from build123d import *

# Parameters (mm, degrees)
F0_R     = 1.5
F1_DEPTH = 13
F0_W     = 7.7
F0_H     = 40
F2_DEPTH = 15
F3_R     = 1.5
F4_DEPTH = 15.001
F5_DEPTH = 5
F6_SIZE  = 1.5


with BuildPart() as f1:
    # F0 (on Right) → F1 (new body)
    with BuildSketch(Plane.YZ):
        Polygon((0, 50), (0, 0), (15, 0), (15, 10), (7.3, 10), (7.3, 50), align=None)
        with Locations((7.5, 5)):
            Circle(F0_R, mode=Mode.SUBTRACT)
    extrude(amount=F1_DEPTH)

    # F0 (on Right) → F2 (join)
    with BuildSketch(Plane.YZ):
        Polygon((0, 50), (0, 0), (15, 0), (15, 10), (7.3, 10), (7.3, 50), align=None)
        with Locations((7.5, 5)):
            Circle(F0_R, mode=Mode.SUBTRACT)
        with Locations((11.15, 30)):
            Rectangle(F0_W, F0_H)
        with Locations((7.5, 5)):
            Circle(F0_R)
    extrude(amount=-F2_DEPTH)

    # F3 (on face) → F4 (cut, through all)
    with BuildSketch(Plane.XZ):
        with Locations((-10, 45)):
            Circle(F3_R)
        with Locations((-10, 5)):
            Circle(F3_R)
    extrude(amount=-F4_DEPTH, mode=Mode.SUBTRACT)

    # F3 (on face) → F5 (cut, symmetric)
    with BuildSketch(Plane.XZ):
        Polygon((-10.010564, 2.401945), (-7.7553, 3.691824), (-7.744737, 6.289879), (-9.989436, 7.598055), (-12.2447, 6.308176), (-12.255263, 3.710121), align=None)
        with Locations((-10, 5)):
            Circle(F3_R, mode=Mode.SUBTRACT)
        Polygon((-7.758047, 46.312877), (-10.016008, 47.598027), (-12.257961, 46.28515), (-12.241953, 43.687123), (-9.983992, 42.401973), (-7.742039, 43.71485), align=None)
        with Locations((-10, 45)):
            Circle(F3_R, mode=Mode.SUBTRACT)
    extrude(amount=F5_DEPTH, both=True, mode=Mode.SUBTRACT)

    # F6
    f6_edges = [f1.edges().sort_by_distance(p)[0] for p in [
        (-15, 0, 25),
        (-1, 0, 50),
        (13, 0, 25),
        (-15, 7.5, 50),
        (-15, 7.5, 0),
        (-1, 0, 0),
        (13, 7.5, 0),
        (13, 3.65, 50),
        (13, 15, 5),
    ]]
    chamfer(f6_edges, length=F6_SIZE)


solid = f1.part
Input: part model. Units: mm. Frame: model coordinates. A direction names the side the tool comes from. Give positions to 0.01 mm unless a question says otherwise; leave off trailing zeros. Loops run counter-clockwise (first coordinate to the right, second up) from the corner with the lowest first, then second, coordinate; pieces in that order, holes last. Notation, with made-up numbers: M 81,54.25 L 126,54.25 A34 cw 126,87.25 Z; hole C 38.25,23 d6. An arc over 180 degrees is marked long. Use one line per item in the form item = value.
1. First-contact query: pin 1 (3 mm diameter, centred on x = 6.5, z = 28.5, fed in from +Y); pin 2 (3 mm diameter, centred on y = 12.5, z = 23.5, fed in from +X). Flat tips, straight axial feed; report the tip coordinate or a pass-through.
Numbers:
pin_1 = 7.3
pin_2 = 0
2. Section query D-D, the plane y = 2.5. Return the cut outline in (x, z), and give its area (3 significant figures).
Numbers:
outline = M -15,1.5 L -13.5,0 L 11.5,0 L 13,1.5 L 13,48.5 L 11.5,50 L -13.5,50 L -15,48.5 Z; hole M -12.26,3.71 L -10.01,2.4 L -7.76,3.69 L -7.74,6.29 L -9.99,7.6 L -12.24,6.31 Z; hole M -12.26,46.29 L -12.24,43.69 L -9.98,42.4 L -7.74,43.71 L -7.76,46.31 L -10.02,47.6 Z
area = 1,360 mm²
3. Section query A-A, the plane y = 10.75. Return the cut outline in (x, z), and give its area (3 significant figures).
Numbers:
outline = M -15,1.5 L -13.5,0 L 11.5,0 L 13,1.5 L 13,10 L 0,10 L 0,50 L -13.5,50 L -15,48.5 Z; hole C -10,5 d3; hole C -10,45 d3
area = 862 mm²
4. Line query: L1, parallel to Z at x = -10, y = 10.5; L2, parallel to Z at x = -11, y = 1.25; L3, parallel to X at y = 12.25, z = 40. Output: solid intervals per line, ascending.
Numbers:
L1 = 0 to 3.5, 6.5 to 43.5, 46.5 to 50
L2 = 0.25 to 2.98, 7.02 to 42.98, 47.02 to 49.75
L3 = -15 to 0
5. Section query C-C, the plane z = 34. Return the cut outline in (x, y), and give its area (3 significant figures).
Numbers:
outline = M -15,1.5 L -13.5,0 L 11.5,0 L 13,1.5 L 13,7.3 L 0,7.3 L 0,15 L -15,15 Z
area = 318 mm²
6. Reachability of faces 1 (the face through (-8.871, 2.465, 46.946)), 2 (the face through (6, 7.3, 30)), 3 (the face through (0, 7, 5)) from +Z, -Z, +X, -X, +Y, -Y: full face, straight path, thin tool, end or side. Return the list, or none.
Numbers:
face_1 = -Y
face_2 = +Z, +X, +Y
face_3 = +X
7. Section query B-B, the plane z = 45. Return the cut outline in (x, y), and give its area (3 significant figures).
Numbers:
outline = M -15,1.5 L -13.5,0 L -12.25,0 L -12.25,5 L -11.5,5 L -11.5,15 L -15,15 Z; M -8.5,5 L -7.75,5 L -7.75,0 L 11.5,0 L 13,1.5 L 13,7.3 L 0,7.3 L 0,15 L -8.5,15 Z
area = 265 mm²
8. Pull-direction query (Z, two-part tool) for faces 4 (the face through (12, 1, 49)), 5 (the face through (-14.2, 8.2, 0.7)), 6 (the face through (-12, 5, 45)); classes: released by +Z, released by -Z, zero draft, split by the parting line, or undercut.
Numbers:
face_4 = released by +Z
face_5 = released by -Z
face_6 = undercut
